```python
from build123d import *

# Parameters (mm, degrees)
F0_W     = 558.8
F0_H     = 101.6
F1_DEPTH = 101.6
F2_R     = 12.7
F3_DEPTH = 101.601


with BuildPart() as f1:
    # F0 (on Top) → F1 (new body)
    with BuildSketch(Plane.XY):
        with Locations((279.4, 50.8)):
            Rectangle(F0_W, F0_H)
    extrude(amount=-F1_DEPTH)

    # F2 (on face) → F3 (cut, through all)
    with BuildSketch(Plane.XY):
        with BuildLine():
            ThreePointArc((127, 38.1), (135.980256, 41.819744), (139.7, 50.8))
            ThreePointArc((139.7, 50.8), (135.980256, 59.780256), (127, 63.5))
            ThreePointArc((127, 63.5), (118.019744, 59.780256), (114.3, 50.8))
            ThreePointArc((114.3, 50.8), (118.019744, 41.819744), (127, 38.1))
        make_face()
        with Locations((431.8, 50.8)):
            Circle(F2_R)
    extrude(amount=-F3_DEPTH, mode=Mode.SUBTRACT)


solid = f1.part
```
Source: CAD feature listing. Evaluate the final solid. Frame: model axes, mm. Round coordinates to 2 decimals unless told otherwise and drop trailing zeros. Loops run counter-clockwise (first coordinate to the right, second up) from the corner with the lowest first, then second, coordinate; pieces in that order, holes last.
1. Contact query for a flat-ended pin moving along its axis: pin 1 (23 mm diameter, centred on x = 431.8, y = 50.8, fed in from -Z). Output: stop coordinate, or through.
2. Section query B-B on z = -82. Output: boundary loops of the cut face in (x, y), and give its area (3 significant figures).
3. Ray query, L1, parallel to X at y = 50, z = -59; L2, parallel to X at y = 52.5, z = -39.5; L3, parallel to Y at x = 431, z = -27. Return the intervals inside material, ascending.
4. Mould query, pull axis X, two halves, no side actions, for faces 1 (the flat face through (0, 50, -50)), 2 (the cylindrical face through (421.7, 43.1, -50.1)), 3 (the flat face through (275, 101.6, -50)), 4 (the flat face through (558.8, 50, -50)). Classes: released by +X, released by -X, zero draft, split by the parting line, or undercut.
5. Section query A-A on x = 431.8. Output: boundary loops of the cut face in (y, z), and give its area (3 significant figures).
Answers below:
1. pin 1: passes through
2. outline: (0, 0) - (558.8, 0) - (558.8, 101.6) - (0, 101.6) - close; hole circle Ø25.4 at (127, 50.8); hole circle Ø25.4 at (431.8, 50.8)
2. area: 55,800 mm2
3. L1: x = 0 to 114.33, 139.67 to 419.13, 444.47 to 558.8
3. L2: x = 0 to 114.41, 139.59 to 419.21, 444.39 to 558.8
3. L3: y = 0 to 38.13, 63.47 to 101.6
4. face 1: released by -X
4. face 2: undercut
4. face 3: zero draft
4. face 4: released by +X
5. outline: (0, -101.6) - (38.1, -101.6) - (38.1, 0) - (0, 0) - close; (63.5, -101.6) - (101.6, -101.6) - (101.6, 0) - (63.5, 0) - close
5. area: 7,740 mm2
